```python
from build123d import *

# Parameters (mm, degrees)
SKETCH1_R           = 1.5
SKETCH1_W           = 26.2015327
SKETCH1_H           = 1
BOSS_EXTRUDE1_DEPTH = 1.5
SKETCH1_3_R         = 1.5
BOSS_EXTRUDE2_DEPTH = 6


with BuildPart() as part:
    # Sketch1 → Boss-Extrude1 (new body)
    with BuildSketch(Plane.XY):
        with BuildLine():
            ThreePointArc((-17.05, 16.75), (-16.317766953, 18.517766953), (-14.55, 19.25))
            Line((-14.55, 19.25), (14.55, 19.25))
            ThreePointArc((14.55, 19.25), (16.317766953, 18.517766953), (17.05, 16.75))
            Line((17.05, 16.75), (17.05, -16.75))
            ThreePointArc((17.05, -16.75), (16.317766953, -18.517766953), (14.55, -19.25))
            Line((14.55, -19.25), (-14.55, -19.25))
            ThreePointArc((-14.55, -19.25), (-16.317766953, -18.517766953), (-17.05, -16.75))
            Line((-17.05, -16.75), (-17.05, 16.75))
        make_face()
        with BuildLine():
            Line((-14.55, -18.4), (14.55, -18.4))
            ThreePointArc((14.55, -18.4), (15.716726189, -17.916726189), (16.2, -16.75))
            Line((16.2, -16.75), (16.2, 16.75))
            ThreePointArc((16.2, 16.75), (15.716726189, 17.916726189), (14.55, 18.4))
            Line((14.55, 18.4), (-14.55, 18.4))
            ThreePointArc((-14.55, 18.4), (-15.716726189, 17.916726189), (-16.2, 16.75))
            Line((-16.2, 16.75), (-16.2, -16.75))
            ThreePointArc((-16.2, -16.75), (-15.716726189, -17.916726189), (-14.55, -18.4))
        make_face(mode=Mode.SUBTRACT)
        with BuildLine():
            Line((-16.2, 16.75), (-16.2, -16.75))
            ThreePointArc((-16.2, -16.75), (-15.716726189, -17.916726189), (-14.55, -18.4))
            Line((-14.55, -18.4), (-13.10076635, -18.4))
            Line((-13.10076635, -18.4), (-13.10076635, -17.4))
            Line((-13.10076635, -17.4), (-14.55, -17.4))
            ThreePointArc((-14.55, -17.4), (-15.009619408, -17.209619408), (-15.2, -16.75))
            Line((-15.2, -16.75), (-15.2, 16.75))
            ThreePointArc((-15.2, 16.75), (-15.009619408, 17.209619408), (-14.55, 17.4))
            Line((-14.55, 17.4), (14.55, 17.4))
            ThreePointArc((14.55, 17.4), (15.009619408, 17.209619408), (15.2, 16.75))
            Line((15.2, 16.75), (15.2, -16.75))
            ThreePointArc((15.2, -16.75), (15.009619408, -17.209619408), (14.55, -17.4))
            Line((14.55, -17.4), (13.10076635, -17.4))
            Line((13.10076635, -17.4), (13.10076635, -18.4))
            Line((13.10076635, -18.4), (14.55, -18.4))
            ThreePointArc((14.55, -18.4), (15.716726189, -17.916726189), (16.2, -16.75))
            Line((16.2, -16.75), (16.2, 16.75))
            ThreePointArc((16.2, 16.75), (15.716726189, 17.916726189), (14.55, 18.4))
            Line((14.55, 18.4), (-14.55, 18.4))
            ThreePointArc((-14.55, 18.4), (-15.716726189, 17.916726189), (-16.2, 16.75))
        make_face()
        with BuildLine():
            ThreePointArc((-14.55, -17.4), (-15.009619408, -17.209619408), (-15.2, -16.75))
            Line((-15.2, -16.75), (-15.2, 16.75))
            ThreePointArc((-15.2, 16.75), (-15.009619408, 17.209619408), (-14.55, 17.4))
            Line((-14.55, 17.4), (14.55, 17.4))
            ThreePointArc((14.55, 17.4), (15.009619408, 17.209619408), (15.2, 16.75))
            Line((15.2, 16.75), (15.2, -16.75))
            ThreePointArc((15.2, -16.75), (15.009619408, -17.209619408), (14.55, -17.4))
            Line((14.55, -17.4), (-14.55, -17.4))
        make_face()
        with Locations((10.05, 14)):
            Circle(SKETCH1_R, mode=Mode.SUBTRACT)
        with Locations((-10.05, 14)):
            Circle(SKETCH1_R, mode=Mode.SUBTRACT)
        with Locations((10.05, -14)):
            Circle(SKETCH1_R, mode=Mode.SUBTRACT)
        with Locations((-10.05, -14)):
            Circle(SKETCH1_R, mode=Mode.SUBTRACT)
        with Locations((10.05, -14)):
            Circle(SKETCH1_R)
        with Locations((10.05, 14)):
            Circle(SKETCH1_R)
        with Locations((-10.05, -14)):
            Circle(SKETCH1_R)
        with Locations((-10.05, 14)):
            Circle(SKETCH1_R)
        with Locations((0, -17.9)):
            Rectangle(SKETCH1_W, SKETCH1_H)
    extrude(amount=BOSS_EXTRUDE1_DEPTH)

    # Sketch1_3 → Boss-Extrude2 (add)
    with BuildSketch(Plane.XY):
        with BuildLine():
            Line((-16.2, 16.75), (-16.2, -16.75))
            ThreePointArc((-16.2, -16.75), (-15.716726189, -17.916726189), (-14.55, -18.4))
            Line((-14.55, -18.4), (-13.10076635, -18.4))
            Line((-13.10076635, -18.4), (-13.10076635, -17.4))
            Line((-13.10076635, -17.4), (-14.55, -17.4))
            ThreePointArc((-14.55, -17.4), (-15.009619408, -17.209619408), (-15.2, -16.75))
            Line((-15.2, -16.75), (-15.2, 16.75))
            ThreePointArc((-15.2, 16.75), (-15.009619408, 17.209619408), (-14.55, 17.4))
            Line((-14.55, 17.4), (14.55, 17.4))
            ThreePointArc((14.55, 17.4), (15.009619408, 17.209619408), (15.2, 16.75))
            Line((15.2, 16.75), (15.2, -16.75))
            ThreePointArc((15.2, -16.75), (15.009619408, -17.209619408), (14.55, -17.4))
            Line((14.55, -17.4), (13.10076635, -17.4))
            Line((13.10076635, -17.4), (13.10076635, -18.4))
            Line((13.10076635, -18.4), (14.55, -18.4))
            ThreePointArc((14.55, -18.4), (15.716726189, -17.916726189), (16.2, -16.75))
            Line((16.2, -16.75), (16.2, 16.75))
            ThreePointArc((16.2, 16.75), (15.716726189, 17.916726189), (14.55, 18.4))
            Line((14.55, 18.4), (-14.55, 18.4))
            ThreePointArc((-14.55, 18.4), (-15.716726189, 17.916726189), (-16.2, 16.75))
        make_face()
        with Locations((-10.05, 14)):
            Circle(SKETCH1_3_R)
        with Locations((-10.05, -14)):
            Circle(SKETCH1_3_R)
        with Locations((10.05, -14)):
            Circle(SKETCH1_3_R)
        with Locations((10.05, 14)):
            Circle(SKETCH1_3_R)
    extrude(amount=BOSS_EXTRUDE2_DEPTH)


solid = part.part
```
Work out the finished part from the listing and answer in its coordinate system (mm). A direction names the side the tool comes from. Round coordinates to 2 decimals unless told otherwise and drop trailing zeros. Write each loop counter-clockwise with the first axis right and the second up, starting at its lowest first coordinate (ties: lowest second). Pieces come first, ordered by that corner, then holes.
1) A cutting plane is placed at B-B on y = -4. Determine the outline of the cut face in (x, z), and give its area (4 significant figures).
2) A cutting plane is placed at A-A on z = 2.9. Determine the outline of the cut face in (x, y), and give its area (3 significant figures).
3) Consider probe 1 along X at (y, z) = (-7, 2.95); probe 2 along X at (y, z) = (-13, 5.45); probe 3 along Y at (x, z) = (-8, 3.6). Determine where each line is inside the solid, lowest interval first.
4) A cutting plane is placed at C-C on x = 10.05. Determine the outline of the cut face in (y, z), and give its area (4 significant figures).
5) Flat-ended cylindrical pins translate along their axes: P1, Ø8, axis at x = 10.5, y = 0, coming from the +Z side; P2, Ø1.6, axis at x = 14, z = 3, coming from the +Y side; P3, Ø1.5, axis at y = -3, z = 5, coming from the +X side. Find the tip coordinate at first contact, or state that the pin passes through.
6) Determine the mould class of faces 1 (the face through (0, 19.25, 1)), 2 (the face through (17.05, 0, 1)), 3 (the face through (0, 17.4, 4)), 4 (the face through (14, -17.4, 4)) for opening direction Y: pulls with the +Y half, pulls with the -Y half, needs draft (parallel to the pull), parting line crosses it, or undercut.
7) Which of the six approach directions +Z, -Z, +X, -X, +Y, -Y give full straight-line access (tool end or side, diameter ignored) to faces 5 (the face through (-15.704, 17.929, 3.718)), 6 (the face through (16.2, 0, 4)), 7 (the face through (14, -18.4, 4))?
8) A cutting plane is placed at D-D on y = 14. Determine the outline of the cut face in (x, z).
Entries:
1. outline: (-17.05, 0) - (17.05, 0) - (17.05, 1.5) - (16.2, 1.5) - (16.2, 6) - (15.2, 6) - (15.2, 1.5) - (-15.2, 1.5) - (-15.2, 6) - (-16.2, 6) - (-16.2, 1.5) - (-17.05, 1.5) - close
1. area: 60.15 mm2
2. outline: (-16.2, -16.75) arc R1.65 ccw to (-14.55, -18.4) - (-13.1, -18.4) - (-13.1, -17.4) - (-14.55, -17.4) arc R0.65 cw to (-15.2, -16.75) - (-15.2, 16.75) arc R0.65 cw to (-14.55, 17.4) - (14.55, 17.4) arc R0.65 cw to (15.2, 16.75) - (15.2, -16.75) arc R0.65 cw to (14.55, -17.4) - (13.1, -17.4) - (13.1, -18.4) - (14.55, -18.4) arc R1.65 ccw to (16.2, -16.75) - (16.2, 16.75) arc R1.65 ccw to (14.55, 18.4) - (-14.55, 18.4) arc R1.65 ccw to (-16.2, 16.75) - close; circle Ø3 at (-10.05, -14); circle Ø3 at (-10.05, 14); circle Ø3 at (10.05, -14); circle Ø3 at (10.05, 14)
2. area: 134 mm2
3. probe 1: x = -16.2 to -15.2, 15.2 to 16.2
3. probe 2: x = -16.2 to -15.2, -11.17 to -8.93, 8.93 to 11.17, 15.2 to 16.2
3. probe 3: y = 17.4 to 18.4
4. outline: (-19.25, 0) - (19.25, 0) - (19.25, 1.5) - (18.4, 1.5) - (18.4, 6) - (17.4, 6) - (17.4, 1.5) - (15.5, 1.5) - (15.5, 6) - (12.5, 6) - (12.5, 1.5) - (-12.5, 1.5) - (-12.5, 6) - (-15.5, 6) - (-15.5, 1.5) - (-19.25, 1.5) - close
4. area: 89.25 mm2
5. P1: stops at z = 1.5
5. P2: stops at y = 18.4
5. P3: stops at x = 16.2
6. face 1: pulls with the +Y half
6. face 2: needs draft
6. face 3: undercut
6. face 4: undercut
7. face 5: +Z, -X, +Y
7. face 6: +Z, +X, +Y, -Y
7. face 7: +Z, +X, -X, -Y
8. outline: (-17.05, 0) - (17.05, 0) - (17.05, 1.5) - (16.2, 1.5) - (16.2, 6) - (15.2, 6) - (15.2, 1.5) - (11.55, 1.5) - (11.55, 6) - (8.55, 6) - (8.55, 1.5) - (-8.55, 1.5) - (-8.55, 6) - (-11.55, 6) - (-11.55, 1.5) - (-15.2, 1.5) - (-15.2, 6) - (-16.2, 6) - (-16.2, 1.5) - (-17.05, 1.5) - close
